```python
from build123d import *

# Parameters (mm, degrees)
F0_R     = 6.35
F1_DEPTH = 19.05
F2_R     = 7.62
F3_DEPTH = 1.27
F4_R     = 4.445
F5_DEPTH = 6.35


with BuildPart() as f1:
    # F0 (on Front) → F1 (new body)
    with BuildSketch(Plane.XZ):
        Circle(F0_R)
    extrude(amount=F1_DEPTH)

    # F2 (on face) → F3 (join)
    with BuildSketch(Plane(origin=(0, 0, 0), x_dir=(-1, 0, 0), z_dir=(0, 1, 0))):
        Circle(F2_R)
    extrude(amount=F3_DEPTH)

    # F4 (on face) → F5 (join)
    with BuildSketch(Plane.XZ.offset(19.05)):
        Circle(F4_R)
    extrude(amount=F5_DEPTH)


solid = f1.part
```
Geometry check sheet. Reference: the model listing, model coordinates, mm. A direction names the side the tool comes from. Round coordinates to 2 decimals unless told otherwise and drop trailing zeros. Loops run counter-clockwise (first coordinate to the right, second up) from the corner with the lowest first, then second, coordinate; pieces in that order, holes last. Notation, with made-up numbers: (0.25, 63.5) - (57.25, 63.5) arc R29 ccw to (57.25, 91.5) - close; hole circle Ø11 at (-34.75, 40). An arc over 180 degrees is marked (long way). Write each question's results on one line, items separated by ' | '. Start each with the question number.
Q1. Cross-section at B-B on x = 0. Enter the section's corners in (y, z) (3 decimals), and give its area (3 significant figures).
Q2. Gauge pin test, flat ends, axial feed: P1, Ø1, axis at x = -4, y = -3, coming from the +Z side; P2, Ø3, axis at x = -2.5, y = -7.5, coming from the +Z side; P3, Ø8, axis at x = -5, y = -10.5, coming from the -Z side. Record the tip position at first contact, or that the pin passes through.
Q3. Cross-section at C-C on y = -23.5. Enter the section's corners in (x, z) (3 decimals).
Q4. Thickness scan on line 1 (Y direction, x = 5.5, z = -4.5); line 2 (Y direction, x = -1, z = -5.5); line 3 (Z direction, x = -3, y = -20.5). Record the ranges inside material, lowest first. Write a range as [from, to].
Q5. Access from +Z, -Z, +X, -X, +Y, -Y to the whole of each face (thin tool, end or side, straight path). Record for faces 1 (the flat face through (3, -19.05, -4)), 2 (the cylindrical face through (1.65, 0.63, -7.44)).
Q6. Cross-section at D-D on x = 6. Enter the section's corners in (y, z), and give its area (3 significant figures).
Q7. Cross-section at A-A on z = 0. Enter the section's corners in (x, y) (3 decimals).
Answers below:
1) outline: (-25.4, -4.445) - (-19.05, -4.445) - (-19.05, -6.35) - (0, -6.35) - (0, -7.62) - (1.27, -7.62) - (1.27, 7.62) - (0, 7.62) - (0, 6.35) - (-19.05, 6.35) - (-19.05, 4.445) - (-25.4, 4.445) - close | area: 318 mm²
2) P1: stops at z = 5.3 | P2: stops at z = 6.27 | P3: stops at z = -6.27
3) outline: circle Ø8.89 at (0, 0)
4) line 1: y = [0, 1.27] | line 2: y = [-19.05, 1.27] | line 3: z = [-3.28, 3.28]
5) face 1: -Y | face 2: +Y, -Y
6) outline: (-19.05, -2.08) - (0, -2.08) - (0, -4.7) - (1.27, -4.7) - (1.27, 4.7) - (0, 4.7) - (0, 2.08) - (-19.05, 2.08) - close | area: 91.1 mm²
7) outline: (-7.62, 0) - (-6.35, 0) - (-6.35, -19.05) - (-4.445, -19.05) - (-4.445, -25.4) - (4.445, -25.4) - (4.445, -19.05) - (6.35, -19.05) - (6.35, 0) - (7.62, 0) - (7.62, 1.27) - (-7.62, 1.27) - close
